The model under review builds one solid part; all positions refer to its coordinate system, in mm. Face numbers are marked on the shaded views. A direction names the side the tool comes from. Give positions to 0.01 mm unless a question says otherwise; leave off trailing zeros. Loops run counter-clockwise (first coordinate to the right, second up) from the corner with the lowest first, then second, coordinate; pieces in that order, holes last. Notation, with made-up numbers: M 39,63.25 L 69,63.25 A26 ccw 69,82.25 Z; hole C 31.25,34.5 d5. An arc over 180 degrees is marked long. Put each result on its own line as item: value. Start each with the question number.
from build123d import *

# Parameters (mm, degrees)
SKETCH_1_W          = 85
SKETCH_1_H          = 15
EXTRUDE_1_DEPTH     = 30
SKETCH_2_R          = 1.4
CUT_EXTRUDE_1_DEPTH = 40
CUT_EXTRUDE_2_DEPTH = 40
FILLET_1_R          = 4
SKETCH_5_R          = 1.8
CUT_EXTRUDE_3_DEPTH = 5
CHAMFER_1_SIZE      = 0.5
CUT_EXTRUDE_4_DEPTH = 24
FILLET_3_R          = 4
CUT_EXTRUDE_START   = -5
SKETCH_9_R          = 1.8
CUT_EXTRUDE_5_DEPTH = 5
FILLET_4_R          = 2


with BuildPart() as part:
    # 草图1 → 凸台-拉伸1 (new body)
    with BuildSketch(Plane(origin=(0, 0, 0), x_dir=(1, 0, 0), z_dir=(0, 1, 0))):
        Rectangle(SKETCH_1_W, SKETCH_1_H)
    extrude(amount=EXTRUDE_1_DEPTH)

    # 草图2 → 切除-拉伸1 (cut)
    with BuildSketch(Plane.XY.offset(7.5)):
        with Locations((-35, 24)):
            Circle(SKETCH_2_R)
        with Locations((35, 24)):
            Circle(SKETCH_2_R)
        with Locations((28, 4.255699158)):
            Circle(SKETCH_2_R)
        with Locations((-28, 4.255699158)):
            Circle(SKETCH_2_R)
    extrude(amount=-CUT_EXTRUDE_1_DEPTH, mode=Mode.SUBTRACT)

    # 草图3 → 切除-拉伸2 (cut)
    with BuildSketch(Plane.XY.offset(7.5)):
        Polygon((-27, 24), (27, 24), (21, 4.255699158), (-21, 4.255699158), align=None)
    extrude(amount=-CUT_EXTRUDE_2_DEPTH, mode=Mode.SUBTRACT)

    # 圆角1
    fillet_1_edges = [part.edges().sort_by_distance(p)[0] for p in [
        (-21, 4.255699158, 0),
        (-27, 24, 0),
        (27, 24, 0),
        (21, 4.255699158, 0),
    ]]
    fillet(fillet_1_edges, radius=FILLET_1_R)

    # 草图5 → 切除-拉伸3 (cut)
    with BuildSketch(Plane(origin=(0, 30, 0), x_dir=(1, 0, 0), z_dir=(0, 1, 0))):
        with Locations(Location((-35, 4.5, 0), (0, 0, 270))):
            Circle(SKETCH_5_R)
        with Locations(Location((35, 4.5, 0), (0, 0, 270))):
            Circle(SKETCH_5_R)
        with Locations(Location((-20, -4.5, 0), (0, 0, 270))):
            Circle(SKETCH_5_R)
        with Locations(Location((20, -4.5, 0), (0, 0, 270))):
            Circle(SKETCH_5_R)
    extrude(amount=-CUT_EXTRUDE_3_DEPTH, mode=Mode.SUBTRACT)

    # 倒角1
    chamfer_1_edges = [part.edges().sort_by_distance(p)[0] for p in [
        (-42.5, 30, 0),
        (42.5, 30, 0),
        (-42.5, 0, 0),
        (42.5, 0, 0),
    ]]
    chamfer(chamfer_1_edges, length=CHAMFER_1_SIZE)

    # 草图6 → 切除-拉伸4 (cut)
    with BuildSketch(Plane.XY.offset(7.5)):
        Polygon((-42.5, 24), (-39.5, 24), (-33.5, 4.255699158), (-42.5, 4.255699158), align=None)
        Polygon((42.5, 24), (42.5, 4.255699158), (33.5, 4.255699158), (39.5, 24), align=None)
    extrude(amount=-CUT_EXTRUDE_4_DEPTH, mode=Mode.SUBTRACT)

    # 圆角3
    fillet_3_edges = [part.edges().sort_by_distance(p)[0] for p in [
        (-39.5, 24, 0),
        (39.5, 24, 0),
    ]]
    fillet(fillet_3_edges, radius=FILLET_3_R)

    # 草图9 → 切除-拉伸5 (cut)
    with BuildSketch(Plane.XZ.offset(CUT_EXTRUDE_START)):
        with Locations(Location((20, 4.5, 0), (0, 0, 90))):
            Circle(SKETCH_9_R)
        with Locations(Location((-20, 4.5, 0), (0, 0, 90))):
            Circle(SKETCH_9_R)
        with Locations(Location((-35, -4.5, 0), (0, 0, 90))):
            Circle(SKETCH_9_R)
        with Locations(Location((35, -4.5, 0), (0, 0, 90))):
            Circle(SKETCH_9_R)
    extrude(amount=CUT_EXTRUDE_5_DEPTH, mode=Mode.SUBTRACT)

    # 圆角4
    # the kernel refuses this fillet: 2 mm, written as the material it adds along each edge
    with BuildSketch(Plane(origin=(-33.5, 4.255699158, 7.5), x_dir=(-1, 0, 0), z_dir=(0, 0, -1))) as fillet_4_piece_1_section:
        with BuildLine():
            CenterArc((FILLET_4_R * 1.34903882702, FILLET_4_R), FILLET_4_R, 163.096751643, 106.903248357)
            Line((FILLET_4_R * 0.392241725729, FILLET_4_R * 1.29075643923), (0, 0))
            Line((0, 0), (FILLET_4_R * 1.34903882702, 0))
        make_face()
    fillet_4_piece_1 = extrude(amount=17.750206698, mode=Mode.PRIVATE)
    fillet_4_piece_1 = split(fillet_4_piece_1, bisect_by=Plane(origin=(-34.397620366, 4.568933738, -7.5), z_dir=(0, 0, 1)), keep=Keep.TOP, mode=Mode.PRIVATE)
    fillet_4_piece_1 = fillet_4_piece_1 - Plane(origin=(-35, 4.568933738, -4.5), x_dir=(0, 0, 1), z_dir=(0, 1, 0)) * Cylinder(1.8, 47, mode=Mode.PRIVATE)
    add(fillet_4_piece_1)
    with BuildSketch(Plane(origin=(-33.5, 4.255699158, 7.5), x_dir=(-1, 0, 0), z_dir=(0, 0, -1))) as fillet_4_piece_2_section:
        with BuildLine():
            CenterArc((FILLET_4_R * 1.34903882702, FILLET_4_R), FILLET_4_R, 163.096751643, 106.903248357)
            Line((FILLET_4_R * 0.392241725729, FILLET_4_R * 1.29075643923), (0, 0))
            Line((0, 0), (FILLET_4_R * 1.34903882702, 0))
        make_face()
    fillet_4_piece_2 = extrude(amount=17.750206698, mode=Mode.PRIVATE)
    fillet_4_piece_2 = split(fillet_4_piece_2, bisect_by=Plane(origin=(-34.145110505, 5.458310784, -7.5), z_dir=(0, 0, 1)), keep=Keep.TOP, mode=Mode.PRIVATE)
    fillet_4_piece_2 = split(fillet_4_piece_2, bisect_by=Plane(origin=(-34.145110505, 5, -4.499999953), z_dir=(0, 1, 0)), keep=Keep.TOP, mode=Mode.PRIVATE)
    add(fillet_4_piece_2)
    with BuildSketch(Plane(origin=(33.5, 4.255699158, 7.5), x_dir=(0.2907564392301515, 0.9567971012948373, 0), z_dir=(0, 0, -1))) as fillet_4_piece_3_section:
        with BuildLine():
            CenterArc((FILLET_4_R * 1.34903882702, FILLET_4_R), FILLET_4_R, 163.096751643, 106.903248357)
            Line((FILLET_4_R * 0.392241725729, FILLET_4_R * 1.29075643923), (0, 0))
            Line((0, 0), (FILLET_4_R * 1.34903882702, 0))
        make_face()
    fillet_4_piece_3 = extrude(amount=17.750206698, mode=Mode.PRIVATE)
    fillet_4_piece_3 = split(fillet_4_piece_3, bisect_by=Plane(origin=(34.133275605, 5.45760424, -7.5), z_dir=(0, 0, 1)), keep=Keep.TOP, mode=Mode.PRIVATE)
    fillet_4_piece_3 = fillet_4_piece_3 - Plane(origin=(35, 5.45760424, -4.5), x_dir=(0, 0, 1), z_dir=(0, 1, 0)) * Cylinder(1.8, 47, mode=Mode.PRIVATE)
    add(fillet_4_piece_3)
    with BuildSketch(Plane(origin=(33.5, 4.255699158, 7.5), x_dir=(0.2907564392301515, 0.9567971012948373, 0), z_dir=(0, 0, -1))) as fillet_4_piece_4_section:
        with BuildLine():
            CenterArc((FILLET_4_R * 1.34903882702, FILLET_4_R), FILLET_4_R, 163.096751643, 106.903248357)
            Line((FILLET_4_R * 0.392241725729, FILLET_4_R * 1.29075643923), (0, 0))
            Line((0, 0), (FILLET_4_R * 1.34903882702, 0))
        make_face()
    fillet_4_piece_4 = extrude(amount=17.750206698, mode=Mode.PRIVATE)
    fillet_4_piece_4 = split(fillet_4_piece_4, bisect_by=Plane(origin=(34.145110504, 5.458310885, -7.5), z_dir=(0, 0, 1)), keep=Keep.TOP, mode=Mode.PRIVATE)
    fillet_4_piece_4 = split(fillet_4_piece_4, bisect_by=Plane(origin=(34.145110504, 5, -4.499999944), z_dir=(0, 1, 0)), keep=Keep.TOP, mode=Mode.PRIVATE)
    add(fillet_4_piece_4)


solid = part.part
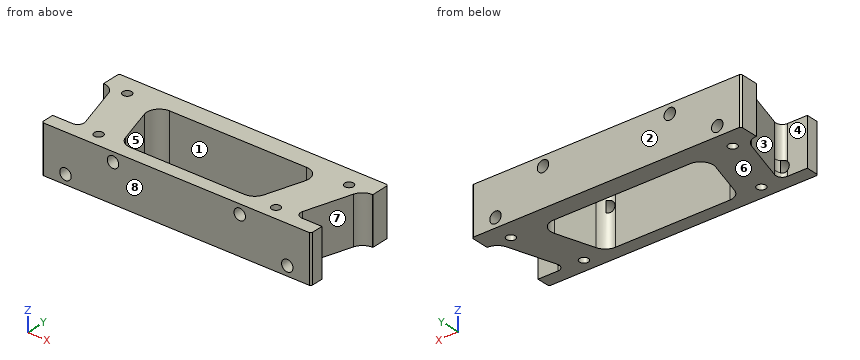
(1) We need section D-D, the plane x = 2. Write out the cut boundary in (y, z).
(2) We need section B-B, the plane y = 26.5. Write out the cut boundary in (x, z).
(3) For the marked faces 4, 5, 6, 7 and 8, list the 3-axis set-ups (+Z, -Z, +X, -X, +Y, -Y) from which the entire face can be reached by the end or side of a thin tool; tool diameter is ignored.
(4) We need section A-A, the plane x = -28. Write out the cut boundary in (y, z), plus the area to 3 significant figures.
(5) Draft analysis for pull direction X (two halves, no side actions). For the marked faces 1, 2 and 3, state which applies: +X half, -X half, draft (parallel to the pull), parting line (faces both ways), or undercut.
(6) We need section C-C, the plane z = -4.5. State how many separate pieces and enclosed holes the cut face has, plus the area to 3 significant figures.
(7) Insertion check: pin 1 (6 mm diameter, centred on x = 35, z = -4.5, fed in from -Y); pin 2 (8 mm diameter, centred on y = 13.5, z = 4.5, fed in from -X); pin 3 (8 mm diameter, centred on y = 17, z = -3.5, fed in from +X); pin 4 (3 mm diameter, centred on x = -35, z = -4.5, fed in from +Y). Each pin has a flat end and moves straight along its axis. Give the tip position at first contact, or say it passes through.
(8) To check wall thickness, follow L1, parallel to X at y = 27.25, z = -4.5; L2, parallel to Z at x = 35, y = 28.75; L3, parallel to Y at x = 28, z = -2. State the ranges of each line that lie inside material, in increasing order. Write a range as [from, to].
Check sheet entries:
1. outline: M 0,-7.5 L 4.26,-7.5 L 4.26,7.5 L 0,7.5 Z; M 24,-7.5 L 30,-7.5 L 30,7.5 L 24,7.5 Z
2. outline: M -42.5,-7.5 L 42.5,-7.5 L 42.5,7.5 L -42.5,7.5 Z; hole C -35,-4.5 d3.6; hole C -20,4.5 d3.6; hole C 20,4.5 d3.6; hole C 35,-4.5 d3.6
3. face 4: +Z, -Z, -X
3. face 5: +Z, -Z
3. face 6: -Z, +X, -X, +Y, -Y
3. face 7: +Z, -Z, +X
3. face 8: +Z, -Z, +X, -X, -Y
4. outline: M 0,-7.5 L 2.86,-7.5 L 2.86,7.5 L 0,7.5 Z; M 5.66,-7.5 L 30,-7.5 L 30,7.5 L 5.66,7.5 Z
4. area: 408 mm²
5. face 1: undercut
5. face 2: draft
5. face 3: -X half
6. separate pieces: 3
6. enclosed holes: 3
6. area: 1,300 mm²
7. pin 1: stops at y = 0
7. pin 2: stops at x = -37.52
7. pin 3: stops at x = 38.59
7. pin 4: stops at y = 25
8. L1: x = [-42.5, -36.8], [-33.2, 33.2], [36.8, 42.5]
8. L2: z = [-7.5, -6.3], [-2.7, 7.5]
8. L3: y = [0, 2.86], [5.66, 30]
